Could you check a few things on this model? Use its own coordinates, in mm. Coordinates: 2 decimals unless noted, no trailing zeros. Loops run counter-clockwise (first coordinate to the right, second up) from the corner with the lowest first, then second, coordinate; pieces in that order, holes last.
from build123d import *

# Parameters (mm, degrees)
SKETCH1_W           = 127
SKETCH1_H           = 127
SKETCH1_W_2         = 121
SKETCH1_H_2         = 121
SKETCH1_R           = 38.5
BOSS_EXTRUDE1_DEPTH = 5
SKETCH3_R           = 45.35
SKETCH3_R_2         = 38.5
BOSS_EXTRUDE2_DEPTH = 3
FILLET1_R           = 6.35
FILLET2_R           = 3.425
SKETCH5_R           = 1.5
CUT_EXTRUDE2_DEPTH  = 90.94164775


with BuildPart() as part:
    # Sketch1 → Boss-Extrude1 (new body)
    # profile 1 of 2: a face of its own
    with BuildSketch(Plane.XY):
        Rectangle(SKETCH1_W, SKETCH1_H)
        Rectangle(SKETCH1_W_2, SKETCH1_H_2, mode=Mode.SUBTRACT)
    # profile 2 of 2: a face of its own
    with BuildSketch(Plane.XY):
        Rectangle(SKETCH1_W_2, SKETCH1_H_2)
        Circle(SKETCH1_R, mode=Mode.SUBTRACT)
    extrude(amount=BOSS_EXTRUDE1_DEPTH)

    # Sketch3 → Boss-Extrude2 (add)
    with BuildSketch(Plane.XY.offset(5)):
        Circle(SKETCH3_R)
        Circle(SKETCH3_R_2, mode=Mode.SUBTRACT)
    extrude(amount=BOSS_EXTRUDE2_DEPTH)

    # Fillet1
    fillet1_edges = [part.edges().sort_by_distance(p)[0] for p in [
        (-63.5, 63.5, 2.5),
        (63.5, 63.5, 2.5),
        (63.5, -63.5, 2.5),
        (-63.5, -63.5, 2.5),
    ]]
    fillet(fillet1_edges, radius=FILLET1_R)

    # Fillet2
    # the kernel refuses this fillet: 3.425 mm, written as the material it takes off along each edge
    with BuildSketch(Plane(origin=(0, 0, 8), x_dir=(1, 0, 0), z_dir=(0, -1, 0))) as fillet2_piece_1:
        with BuildLine():
            CenterArc((41.951470906, -3.425), FILLET2_R, 7.12806839, 82.87193161)
            Line((41.951470906, 0), (41.951470906, 0.0685))
            Line((41.951470906, 0.0685), (45.35, 0.0685))
            Line((45.35, 0.0685), (45.4185, 0))
            ThreePointArc((45.4185, 0), (45.4185, -1.5), (45.417970582, -2.9915))
            Line((45.417970582, -2.9915), (45.35, -3))
        make_face()
    revolve(axis=Axis((0, 0, 8), (0, 0, 1)), mode=Mode.SUBTRACT)

    # Sketch5 → Cut-Extrude2 (cut, through all)
    with BuildSketch(Plane.XY.offset(5)):
        with Locations((-57.15, 57.15)):
            Circle(SKETCH5_R)
        with Locations((-57.15, -57.15)):
            Circle(SKETCH5_R)
        with Locations((57.15, -57.15)):
            Circle(SKETCH5_R)
        with Locations((57.15, 57.15)):
            Circle(SKETCH5_R)
    extrude(amount=-CUT_EXTRUDE2_DEPTH, mode=Mode.SUBTRACT)


solid = part.part
1) Imagine slicing it at B-B on z = 2.5. List the corners of the cut face in (x, y) for me, plus the area to 3 significant figures.
2) If I drill on L1, parallel to Y at x = 0, z = 3; L2, parallel to Y at x = -57.15, z = 1.45; L3, parallel to Y at x = 56, z = 0.75, over which ranges is the centre line in solid material (lowest first)?
3) We'd pull the mould along X, two halves only. Please class faces 1 (the cylindrical face through (-58.26, -56.14, 2.54)), 2 (the cylindrical face through (-57.345, 58.637, 2.535)), 3 (the flat face through (-15, 43, 5)), 4 (the cylindrical face through (-61.59, 61.69, 2.54)): released by +X, released by -X, zero draft, split by the parting line, or undercut.
4) Will these pins go through, and if not, where does the flat tip stop? pin 1 (1.5 mm diameter, centred on y = 37, z = 6, fed in from -X); pin 2 (4 mm diameter, centred on x = 57.15, y = -57.15, fed in from +Z).
5) Imagine slicing it at A-A on y = 0. List the corners of the cut face in (x, z) for me (3 decimals), plus the area to 3 significant figures.
Solved:
1. outline: (-63.5, -57.15) arc R6.35 ccw to (-57.15, -63.5) - (57.15, -63.5) arc R6.35 ccw to (63.5, -57.15) - (63.5, 57.15) arc R6.35 ccw to (57.15, 63.5) - (-57.15, 63.5) arc R6.35 ccw to (-63.5, 57.15) - close; hole circle Ø3 at (-57.15, -57.15); hole circle Ø3 at (-57.15, 57.15); hole circle Ø77 at (0, 0); hole circle Ø3 at (57.15, -57.15); hole circle Ø3 at (57.15, 57.15)
1. area: 11,400 mm2
2. L1: y = -63.5 to -38.5, 38.5 to 63.5
2. L2: y = -63.5 to -58.65, -55.65 to 55.65, 58.65 to 63.5
2. L3: y = -63.5 to -58.11, -56.19 to 56.19, 58.11 to 63.5
3. face 1: undercut
3. face 2: undercut
3. face 3: zero draft
3. face 4: released by -X
4. pin 1: stops at x = -26.89
4. pin 2: stops at z = 5
5. outline: (-63.5, 0) - (-38.5, 0) - (-38.5, 8) - (-41.951, 8) arc R3.425 ccw to (-45.35, 5) - (-63.5, 5) - close; (38.5, 0) - (63.5, 0) - (63.5, 5) - (45.35, 5) arc R3.425 ccw to (41.951, 8) - (38.5, 8) - close
5. area: 286 mm2
